The figure shows three views and two pictorial views of one solid part (mm, origin at its lowest corner). Answer the questions. A direction names the side the tool comes from. Give positions to 0.01 mm unless a question says otherwise; leave off trailing zeros. Write each loop counter-clockwise with the first axis right and the second up, starting at its lowest first coordinate (ties: lowest second). Pieces come first, ordered by that corner, then holes. Notation, with made-up numbers: M 16,43.5 L 72,43.5 A15 cw 72,61.5 Z; hole C 64,44.25 d8. An arc over 180 degrees is marked long. Return JSON: item names as keys, results as strings.
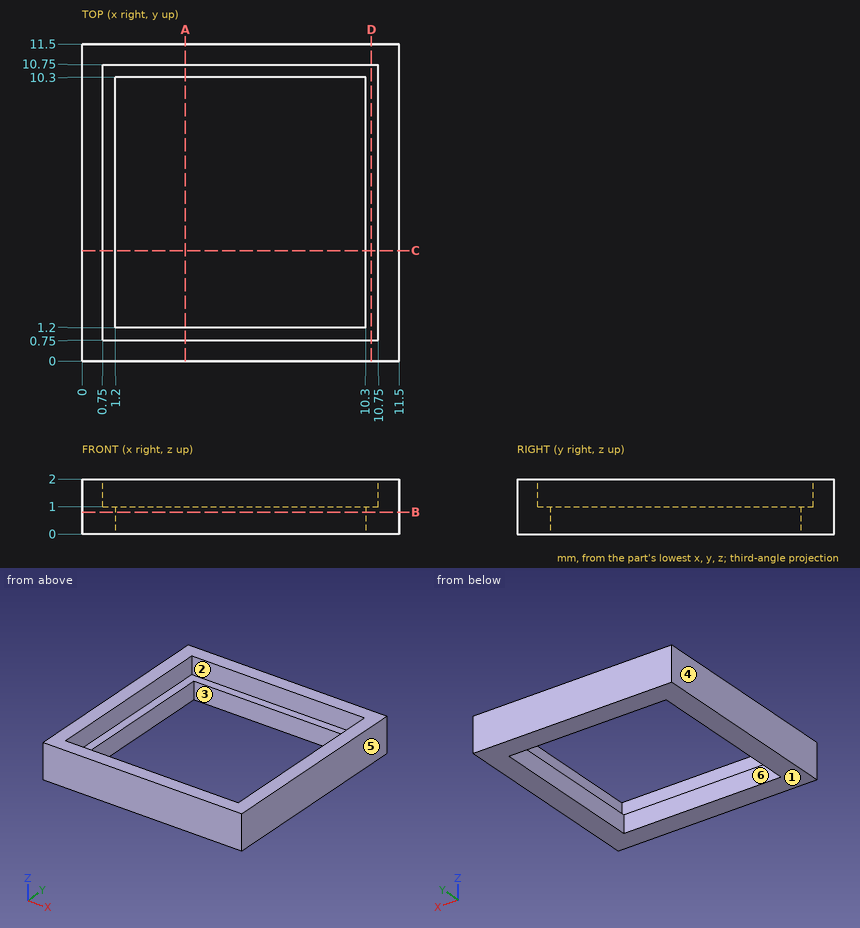
Item 1: Given pin 1 Ø3 at (x, y) = (7, 4.5) entering from +Z, flat-ended and moving along its own axis, determine where the tip first touches the part or whether it passes through.
Geometry results:
{"pin 1": "passes through"}
Item 2: A cutting plane is placed at B-B, the plane z = 0.8. Write down the section's boundary in (x, y).
Geometry results:
{"outline": "M 0,0 L 11.5,0 L 11.5,11.5 L 0,11.5 Z; hole M 1.2,1.2 L 10.3,1.2 L 10.3,10.3 L 1.2,10.3 Z"}
Item 3: Determine the mould class of the marked faces 4, 5 and 6 for opening direction X: +X half, -X half, draft (parallel to the pull), parting line (faces both ways), or undercut.
Geometry results:
{"face 4": "-X half", "face 5": "+X half", "face 6": "undercut"}
Item 4: Find the intervals of material crossed by line 1 (Y direction, x = 7.5, z = 1.15); line 2 (Y direction, x = 4.75, z = 0.5), in increasing order.
Geometry results:
{"line 1": "y = 0 to 0.75, 10.75 to 11.5", "line 2": "y = 0 to 1.2, 10.3 to 11.5"}
Item 5: Which of the six approach directions +Z, -Z, +X, -X, +Y, -Y give full straight-line access (tool end or side, diameter ignored) to the marked faces 1, 2 and 3?
Geometry results:
{"face 1": "-Z, +X, -X, +Y, -Y", "face 2": "+Z", "face 3": "+Z, -Z"}
Item 6: A cutting plane is placed at D-D, the plane x = 10.5. Write down the section's boundary in (y, z).
Geometry results:
{"outline": "M 0,0 L 11.5,0 L 11.5,2 L 10.75,2 L 10.75,1 L 0.75,1 L 0.75,2 L 0,2 Z"}
Item 7: A cutting plane is placed at A-A, the plane x = 3.75. Write down the section's boundary in (y, z).
Geometry results:
{"outline": "M 0,0 L 1.2,0 L 1.2,1 L 0.75,1 L 0.75,2 L 0,2 Z; M 10.3,0 L 11.5,0 L 11.5,2 L 10.75,2 L 10.75,1 L 10.3,1 Z"}
